from build123d import *

# Parameters (mm, degrees)
BOSS_EXTRUDE1_DEPTH = 3
FILLET1_R           = 5
CUT_EXTRUDE8_DEPTH  = 177.164695669


with BuildPart() as part:
    # Sketch1 → Boss-Extrude1 (new body)
    with BuildSketch(Plane.XY):
        Polygon((-75, -145), (75, -145), (75, -55), (100, -55), (100, 55), (75, 55), (75, 145), (-75, 145), (-75, 55), (-100, 55), (-100, -55), (-75, -55), align=None)
    extrude(amount=BOSS_EXTRUDE1_DEPTH)

    # Fillet1
    fillet1_edges = [part.edges().sort_by_distance(p)[0] for p in [
        (-75, -55, 1.5),
        (-100, -55, 1.5),
        (-100, 55, 1.5),
        (-75, 55, 1.5),
        (-75, 145, 1.5),
        (75, 145, 1.5),
        (75, 55, 1.5),
        (100, 55, 1.5),
        (100, -55, 1.5),
        (75, -55, 1.5),
        (75, -145, 1.5),
        (-75, -145, 1.5),
    ]]
    fillet(fillet1_edges, radius=FILLET1_R)

    # Sketch13 → Cut-Extrude8 (cut, through all)
    with BuildSketch(Plane(origin=(0, 0, 0), x_dir=(-1, 0, 0), z_dir=(0, 0, -1))):
        with BuildLine():
            Line((-55, 50), (-42.5, 50))
            ThreePointArc((-42.5, 50), (-35.428932188, 52.928932188), (-32.5, 60))
            Line((-32.5, 60), (-32.5, 65))
            ThreePointArc((-32.5, 65), (-29.571067812, 72.071067812), (-22.5, 75))
            Line((-22.5, 75), (22.5, 75))
            ThreePointArc((22.5, 75), (29.571067812, 72.071067812), (32.5, 65))
            Line((32.5, 65), (32.5, 60))
            ThreePointArc((32.5, 60), (35.428932188, 52.928932188), (42.5, 50))
            Line((42.5, 50), (55, 50))
            ThreePointArc((55, 50), (58.535533906, 48.535533906), (60, 45))
            Line((60, 45), (60, 5))
            ThreePointArc((60, 5), (58.535533906, 1.464466094), (55, 0))
            Line((55, 0), (-55, 0))
            ThreePointArc((-55, 0), (-58.535533906, 1.464466094), (-60, 5))
            Line((-60, 5), (-60, 45))
            ThreePointArc((-60, 45), (-58.535533906, 48.535533906), (-55, 50))
        make_face()
    extrude(amount=-CUT_EXTRUDE8_DEPTH, mode=Mode.SUBTRACT)


solid = part.part
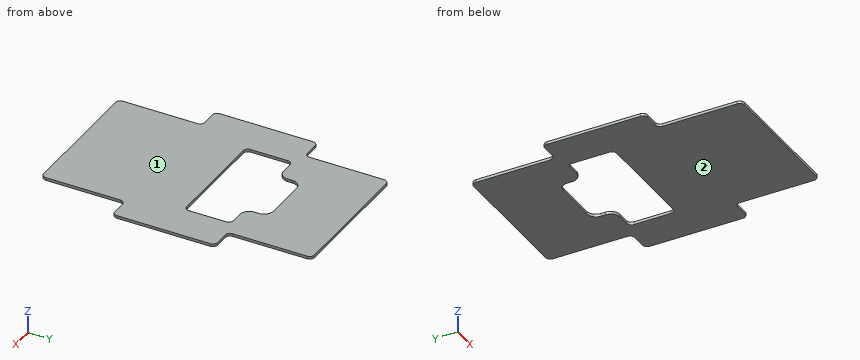
Geometry check sheet. Reference: the model listing, model coordinates, mm. Face numbers are marked on the shaded views. Give positions to 0.01 mm unless a question says otherwise; leave off trailing zeros. Loops run counter-clockwise (first coordinate to the right, second up) from the corner with the lowest first, then second, coordinate; pieces in that order, holes last. Notation, with made-up numbers: (-7.5, 68.5) -> (43.5, 68.5) arc R17 cw to (43.5, 78.5) -> close; hole circle Ø11 at (4.25, -39). An arc over 180 degrees is marked (long way). Answer in a Markdown table with one row per item. Add a question column.
1) Gauge pin test, flat ends, axial feed: P1, Ø1, axis at x = -58, y = 24.5, coming from the +Z side; P2, Ø0.9, axis at x = 86, z = 1.5, coming from the +Y side; P3, Ø1.5, axis at x = 88, z = 1.5, coming from the -Y side; P4, Ø0.9, axis at y = -90, z = 1.5, coming from the +X side. Record the tip position at first contact, or that the pin passes through.
2) Material ranges on probe 1 along Y at (x, z) = (43, 2.3); probe 2 along Y at (x, z) = (-1, 1.6); probe 3 along X at (y, z) = (21.5, 0.45), recorded low to high. Write a range as from..to.
3) Cross-section at D-D on y = -70.5. Record the boundary of the cut face in (x, z).
4) Draft check along Z on the marked faces 1 and 2. Enter one of: pulls with the +Z half, pulls with the -Z half, needs draft (parallel to the pull), parting line crosses it, or undercut.
5) Cross-section at A-A on x = -2. Record the boundary of the cut face in (y, z), and give its area (3 significant figures).
6) Cross-section at C-C on x = -85.5. Record the boundary of the cut face in (y, z), and give its area (3 significant figures).
7) Cross-section at B-B on y = 41. Record the boundary of the cut face in (x, z).
Outcome:
| question | item | result |
|---|---|---|
| 1 | P1 | passes through |
| 1 | P2 | stops at y = 55 |
| 1 | P3 | stops at y = -55 |
| 1 | P4 | stops at x = 75 |
| 2 | probe 1 | y = -145..0, 50..145 |
| 2 | probe 2 | y = -145..0, 75..145 |
| 2 | probe 3 | x = -100..-60, 60..100 |
| 3 | outline | (-75, 0) -> (75, 0) -> (75, 3) -> (-75, 3) -> close |
| 4 | face 1 | pulls with the +Z half |
| 4 | face 2 | pulls with the -Z half |
| 5 | outline | (-145, 0) -> (0, 0) -> (0, 3) -> (-145, 3) -> close; (75, 0) -> (145, 0) -> (145, 3) -> (75, 3) -> close |
| 5 | area | 645 mm^2 |
| 6 | outline | (-55, 0) -> (55, 0) -> (55, 3) -> (-55, 3) -> close |
| 6 | area | 330 mm^2 |
| 7 | outline | (-100, 0) -> (-60, 0) -> (-60, 3) -> (-100, 3) -> close; (60, 0) -> (100, 0) -> (100, 3) -> (60, 3) -> close |
